Input: part model. Units: mm. Frame: model coordinates. A direction names the side the tool comes from. Coordinates: 2 decimals unless noted, no trailing zeros. Loops run counter-clockwise (first coordinate to the right, second up) from the corner with the lowest first, then second, coordinate; pieces in that order, holes last. Notation, with made-up numbers: (51.25, 57.25) - (77.25, 57.25) arc R17 ccw to (77.25, 70.25) - close; hole circle Ø3 at (56, 31.5). An arc over 180 degrees is marked (long way). Use a Markdown table: item, result. Add a question column.
1. Section query A-A on z = -21.25. Return the cut outline in (x, y), then the cut area to 3 significant figures.
2. Access query for faces 1 (the face through (19, 0, -8)), 2 (the face through (30, 5, -12.7)). Directions: +Z, -Z, +X, -X, +Y, -Y. A direction counts if a zero-diameter tool reaches every point of the face in a straight line with its end or side. Return the directions, or none.
3. Section query C-C on x = 16.5. Return the cut outline in (y, z), then the cut area to 3 significant figures.
4. Contact query for flat-ended pins moving along their axis: P1, Ø4, axis at y = 4, z = -15, coming from the +X side; P2, Ø3, axis at x = 27.5, y = 5, coming from the -Z side. Output: stop coordinate, or through.
5. Ray query, L1, parallel to X at y = 9, z = -22.25; L2, parallel to Z at x = 43, y = 9.75; L3, parallel to Z at x = 6, y = 6.75 (3 decimals). Return the intervals inside material, ascending. Write a range as [from, to].
6. Draft query along X for faces 3 (the face through (11.008, 4.93, -26.965)), 4 (the face through (19, 10, -8)), 5 (the face through (1.6, 4.9, -27)), 6 (the face through (5.743, 4.93, -19.776)). Return one class per face: released by +X, released by -X, zero draft, split by the parting line, or undercut.
7. Section query D-D on z = -15.25. Return the cut outline in (x, y).
```python
from build123d import *

# Parameters (mm, degrees)
SKETCH1_R           = 2.50825
BOSS_EXTRUDE1_DEPTH = 10
FILLET1_R           = 3.175
CHAMFER1_SIZE       = 3.175


with BuildPart() as part:
    # Sketch1 → Boss-Extrude1 (new body)
    with BuildSketch(Plane(origin=(0, 0, 0), x_dir=(1, 0, 0), z_dir=(0, 1, 0))):
        with BuildLine():
            Line((0, 28.575), (0, 0))
            Line((0, 0), (47.625, 0))
            ThreePointArc((47.625, 0), (49.87006403, 0.92993597), (50.8, 3.175))
            Line((50.8, 3.175), (50.8, 9.525))
            ThreePointArc((50.8, 9.525), (49.87006403, 11.77006403), (47.625, 12.7))
            Line((47.625, 12.7), (12.573, 12.7))
            Line((12.573, 12.7), (12.573, 28.575))
            Line((12.573, 28.575), (0, 28.575))
        make_face()
        with Locations((6.2865, 22.225)):
            Circle(SKETCH1_R, mode=Mode.SUBTRACT)
    extrude(amount=BOSS_EXTRUDE1_DEPTH)

    # Fillet1
    fillet1_edges = [part.edges().sort_by_distance(p)[0] for p in [
        (0, 5, 0),
    ]]
    fillet(fillet1_edges, radius=FILLET1_R)

    # Chamfer1
    chamfer1_edges = [part.edges().sort_by_distance(p)[0] for p in [
        (12.573, 5, -28.575),
        (0, 5, -28.575),
    ]]
    chamfer(chamfer1_edges, length=CHAMFER1_SIZE)


solid = part.part
```
Resolved:
| question | item | result |
|---|---|---|
| 1 | outline | (0, 0) - (3.98, 0) - (3.98, 10) - (0, 10) - close; (8.6, 0) - (12.57, 0) - (12.57, 10) - (8.6, 10) - close |
| 1 | area | 79.5 mm² |
| 2 | face 1 | +Z, -Z, +X, -X, -Y |
| 2 | face 2 | -Z, +X, +Y, -Y |
| 3 | outline | (0, -12.7) - (10, -12.7) - (10, 0) - (0, 0) - close |
| 3 | area | 127 mm² |
| 4 | P1 | x = 12.57 |
| 4 | P2 | z = -12.7 |
| 5 | L1 | [0, 3.78], [8.79, 12.57] |
| 5 | L2 | [-12.7, 0] |
| 5 | L3 | [-28.575, -24.717], [-19.733, 0] |
| 6 | face 3 | released by +X |
| 6 | face 4 | zero draft |
| 6 | face 5 | released by -X |
| 6 | face 6 | undercut |
| 7 | outline | (0, 0) - (12.57, 0) - (12.57, 10) - (0, 10) - close |
